from build123d import *

# Parameters (mm, degrees)
F0_R     = 2.0193
F1_DEPTH = 3.81
F2_DEPTH = 38.1
F3_R     = 1.89865
F4_DEPTH = 67.311


with BuildPart() as f1:
    # F0 (on Front) → F1 (new body)
    with BuildSketch(Plane.XZ):
        Polygon((0, 0), (0, 19.05), (-57.15, 19.05), (-63.5, 12.7), (-63.5, 0), (-63.5, -12.7), (-57.15, -19.05), (0, -19.05), align=None)
        with Locations((-50.6222, -13.8176)):
            Circle(F0_R, mode=Mode.SUBTRACT)
        with Locations((-21.59, -13.8176)):
            Circle(F0_R, mode=Mode.SUBTRACT)
        with Locations((-50.6222, 13.8176)):
            Circle(F0_R, mode=Mode.SUBTRACT)
        with Locations((-21.59, 13.8176)):
            Circle(F0_R, mode=Mode.SUBTRACT)
    extrude(amount=F1_DEPTH)

    # F0 (on Front) → F2 (join)
    with BuildSketch(Plane.XZ):
        Polygon((3.81, 19.05), (0, 19.05), (0, 0), (0, -19.05), (3.81, -19.05), (3.81, 0), align=None)
    extrude(amount=F2_DEPTH)

    # F3 (on face) → F4 (cut, through all)
    with BuildSketch(Plane.YZ.offset(3.81)):
        with Locations((-22.86, 9.779)):
            Circle(F3_R)
        with Locations((-22.86, -9.779)):
            Circle(F3_R)
        with Locations((-32.639, 0)):
            Circle(F3_R)
        with Locations((-13.081, 0)):
            Circle(F3_R)
    extrude(amount=-F4_DEPTH, mode=Mode.SUBTRACT)


solid = f1.part
Geometry: final body of the model. Coordinates: model frame, mm. A direction names the side the tool comes from. Round coordinates to 2 decimals unless told otherwise and drop trailing zeros. Loops run counter-clockwise (first coordinate to the right, second up) from the corner with the lowest first, then second, coordinate; pieces in that order, holes last. Notation, with made-up numbers: (42.5, 77) -> (46.5, 77) arc R22 ccw to (46.5, 99) -> close; hole circle Ø10 at (48, 84). An arc over 180 degrees is marked (long way). One line per question, with ' | ' between items. Start each with the question number.
1. Mould query, pull axis Z, two halves, no side actions, for faces 3 (the face through (-16, -3, -19.05)), 4 (the face through (1.932, -34.146, -1.155)), 5 (the face through (1.932, -14.978, 0.083)), 6 (the face through (3.81, -19, 0)). Classes: pulls with the +Z half, pulls with the -Z half, needs draft (parallel to the pull), parting line crosses it, or undercut.
2. Set-up query: faces 1 (the face through (2, -38.1, 0)), 2 (the face through (-32, -3.81, 0)). Return all of +Z, -Z, +X, -X, +Y, -Y with unobstructed straight access to the full face (end or side cutting, diameter ignored); none if empty.
3. Section A-A on z = 0. Output: boundary loops of the cut face in (x, y).
4. Section D-D on y = -12. Output: boundary loops of the cut face in (x, z).
5. Contact query for flat-ended pins moving along their axis: pin 1 (4.5 mm diameter, centred on y = -22.86, z = 9.779, fed in from -X); pin 2 (10 mm diameter, centred on x = -8.5, z = 15, fed in from -Y). Output: stop coordinate, or through.
6. Section C-C on x = -21.59. Output: boundary loops of the cut face in (y, z).
7. Line query: line 1 along Z through (x, y) = (2.15, -22.86); line 2 along Z through (x, y) = (-21.59, -1.05); line 3 along X through (y, z) = (-36, 16). Output: solid intervals per line, ascending. Write a range as [from, to].
8. Section B-B on y = -22.86. Output: boundary loops of the cut face in (x, z), and give its area (3 significant figures).
Returned:
1) face 3: pulls with the -Z half | face 4: undercut | face 5: undercut | face 6: needs draft
2) face 1: +Z, -Z, +X, -X, -Y | face 2: +Z, -Z, -X, -Y
3) outline: (-63.5, -3.81) -> (0, -3.81) -> (0, -11.18) -> (3.81, -11.18) -> (3.81, 0) -> (-63.5, 0) -> close; (0, -38.1) -> (3.81, -38.1) -> (3.81, -34.54) -> (0, -34.54) -> close; (0, -30.74) -> (3.81, -30.74) -> (3.81, -14.98) -> (0, -14.98) -> close
4) outline: (0, -19.05) -> (3.81, -19.05) -> (3.81, -1.56) -> (0, -1.56) -> close; (0, 1.56) -> (3.81, 1.56) -> (3.81, 19.05) -> (0, 19.05) -> close
5) pin 1: stops at x = 0 | pin 2: stops at y = -3.81
6) outline: (-3.81, -19.05) -> (0, -19.05) -> (0, -15.84) -> (-3.81, -15.84) -> close; (-3.81, -11.8) -> (0, -11.8) -> (0, 11.8) -> (-3.81, 11.8) -> close; (-3.81, 15.84) -> (0, 15.84) -> (0, 19.05) -> (-3.81, 19.05) -> close
7) line 1: z = [-19.05, -11.68], [-7.88, 7.88], [11.68, 19.05] | line 2: z = [-19.05, -15.84], [-11.8, 11.8], [15.84, 19.05] | line 3: x = [0, 3.81]
8) outline: (0, -19.05) -> (3.81, -19.05) -> (3.81, -11.68) -> (0, -11.68) -> close; (0, -7.88) -> (3.81, -7.88) -> (3.81, 7.88) -> (0, 7.88) -> close; (0, 11.68) -> (3.81, 11.68) -> (3.81, 19.05) -> (0, 19.05) -> close | area: 116 mm2
